The model under review builds one solid part; all positions refer to its coordinate system, in mm. A direction names the side the tool comes from. Round coordinates to 2 decimals unless told otherwise and drop trailing zeros. Write each loop counter-clockwise with the first axis right and the second up, starting at its lowest first coordinate (ties: lowest second). Pieces come first, ordered by that corner, then holes. Notation, with made-up numbers: (3.25, 51) -> (47.25, 51) arc R25 ccw to (47.25, 89) -> close; hole circle Ø11 at (19.5, -7.75). An arc over 180 degrees is marked (long way). Answer as a JSON object with one key per item and string values. Group by question number.
1) We need section D-D, the plane x = 31. Write out the cut boundary in (y, z) (3 decimals), then the cut area to 3 significant figures.
2) We need section C-C, the plane y = 23.5. Write out the cut boundary in (x, z).
3) Mouldability with a two-part tool opening along Y and no side actions: class faces 5 (the flat face through (-25.4, 20, 9)), 6 (the flat face through (0, 38.1, 8)), 7 (the flat face through (0, 22, 8)), 8 (the flat face through (25.4, -11, 8)) as pulls with the +Y half, pulls with the -Y half, needs draft (parallel to the pull), parting line crosses it, or undercut.
4) We need section B-B, the plane x = 14. Write out the cut boundary in (y, z), then the cut area to 3 significant figures.
5) Insertion check: pin 1 Ø4 at (y, z) = (29, 13.5) entering from -X; pin 2 Ø8 at (y, z) = (5, 6) entering from +X; pin 3 Ø5 at (x, y) = (-15, 22) entering from +Z; pin 4 Ø10 at (y, z) = (20.342, 8.5) entering from -X. Each pin has a flat end and moves straight along its axis. Give the tip position at first contact, or say it passes through.
6) We need section A-A, the plane z = 14.75. Write out the cut boundary in (x, y), then the cut area to 3 significant figures.
7) Machinability: for faces 1 (the cylindrical face through (31.84, 13.62, 3.34)), 2 (the cylindrical face through (-31.839, 22.179, 0.227)), 3 (the flat face through (0, -38.1, 8)), 4 (the flat face through (0, 8.161, 13)), which of the approach directions +Z, -Z, +X, -X, +Y, -Y give a long, thin tool a straight path to every point of the face, cutting with its end or side? Answer none if there is none.
8) To check wall thickness, follow probe 1 along Y at (x, z) = (-15.5, 8.5); probe 2 along X at (y, z) = (12, 13.75); probe 3 along Z at (x, y) = (-3, -5). State the ranges of each line that lie inside material, in increasing order. Write a range as [from, to].
from build123d import *

# Parameters (mm, degrees)
F0_W      = 50.8
F0_H      = 76.2
F1_DEPTH  = 17
F3_W      = 44.944652
F3_H      = 27
F4_DEPTH  = 9
F5_R      = 9.5
F6_DEPTH  = 12.7
F7_R      = 8.475
F8_DEPTH  = 12.7
F9_R      = 9.5
F10_DEPTH = 12.7
F11_R     = 8.475
F12_DEPTH = 12.7


with BuildPart() as f1:
    # F0 (on Top) → F1 (new body)
    with BuildSketch(Plane.XY):
        Rectangle(F0_W, F0_H)
    extrude(amount=F1_DEPTH)

    # F3 (on face) → F4 (cut)
    with BuildSketch(Plane.XY.offset(17)):
        with Locations((0, 21.661439)):
            Rectangle(F3_W, F3_H)
    extrude(amount=-F4_DEPTH, mode=Mode.SUBTRACT)

    # F5 (on face) → F6 (join)
    with BuildSketch(Plane.YZ.offset(25.4)):
        with Locations((20.341752, 8.5)):
            Circle(F5_R)
    extrude(amount=F6_DEPTH)

    # F7 (on face) → F8 (cut)
    with BuildSketch(Plane.YZ.offset(38.1)):
        with Locations((20.341752, 8.5)):
            Circle(F7_R)
    extrude(amount=-F8_DEPTH, mode=Mode.SUBTRACT)

    # F9 (on face) → F10 (join)
    with BuildSketch(Plane(origin=(-25.4, 0, 0), x_dir=(0, -1, 0), z_dir=(-1, 0, 0))):
        with Locations((-20.342, 8.5)):
            Circle(F9_R)
    extrude(amount=F10_DEPTH)

    # F11 (on face) → F12 (cut)
    with BuildSketch(Plane(origin=(-38.1, 0, 0), x_dir=(0, -1, 0), z_dir=(-1, 0, 0))):
        with Locations((-20.342, 8.5)):
            Circle(F11_R)
    extrude(amount=-F12_DEPTH, mode=Mode.SUBTRACT)


solid = f1.part
Here are the results:
{
 "1": {"outline": "circle Ø19 at (20.342, 8.5); hole circle Ø16.95 at (20.342, 8.5)", "area": "57.9 mm^2"},
 "2": {"outline": "(-38.1, -0.46) -> (-25.4, -0.46) -> (-25.4, 0) -> (25.4, 0) -> (25.4, -0.46) -> (38.1, -0.46) -> (38.1, 0.64) -> (25.4, 0.64) -> (25.4, 16.36) -> (38.1, 16.36) -> (38.1, 17.46) -> (25.4, 17.46) -> (25.4, 17) -> (22.47, 17) -> (22.47, 8) -> (-22.47, 8) -> (-22.47, 17) -> (-25.4, 17) -> (-25.4, 17.46) -> (-38.1, 17.46) -> (-38.1, 16.36) -> (-25.4, 16.36) -> (-25.4, 0.64) -> (-38.1, 0.64) -> close"},
 "3": {"face 5": "undercut", "face 6": "pulls with the +Y half", "face 7": "undercut", "face 8": "needs draft"},
 "4": {"outline": "(-38.1, 0) -> (38.1, 0) -> (38.1, 17) -> (35.16, 17) -> (35.16, 8) -> (8.16, 8) -> (8.16, 17) -> (-38.1, 17) -> close", "area": "1,050 mm^2"},
 "5": {"pin 1": "stops at x = -38.1", "pin 2": "stops at x = 25.4", "pin 3": "stops at z = 8", "pin 4": "stops at x = -25.4"},
 "6": {"outline": "(-38.1, 13.19) -> (-25.4, 13.19) -> (-25.4, -38.1) -> (25.4, -38.1) -> (25.4, 13.19) -> (38.1, 13.19) -> (38.1, 14.62) -> (25.4, 14.62) -> (25.4, 26.07) -> (38.1, 26.07) -> (38.1, 27.5) -> (25.4, 27.5) -> (25.4, 38.1) -> (-25.4, 38.1) -> (-25.4, 27.5) -> (-38.1, 27.5) -> (-38.1, 26.07) -> (-25.4, 26.07) -> (-25.4, 14.62) -> (-38.1, 14.62) -> close; hole (-22.47, 8.16) -> (22.47, 8.16) -> (22.47, 35.16) -> (-22.47, 35.16) -> close", "area": "2,730 mm^2"},
 "7": {"face 1": "+X", "face 2": "-X", "face 3": "+Z, -Z, +X, -X, -Y", "face 4": "+Z"},
 "8": {"probe 1": "y = [-38.1, 8.16], [35.16, 38.1]", "probe 2": "x = [-25.4, -22.47], [22.47, 25.4]", "probe 3": "z = [0, 17]"}
}
